Could you check a few things on this drawing? It's one solid part, dimensions in mm from its lowest x, y, z. Give positions to 0.01 mm unless a question says otherwise; leave off trailing zeros. Loops run counter-clockwise (first coordinate to the right, second up) from the corner with the lowest first, then second, coordinate; pieces in that order, holes last. Notation, with made-up numbers: (38.25, 69.25) - (66.25, 69.25) arc R8 ccw to (66.25, 74.25) - close; hole circle Ø11 at (66.25, 21.25). An arc over 180 degrees is marked (long way). Answer as a JSON object with one key per item and string values.
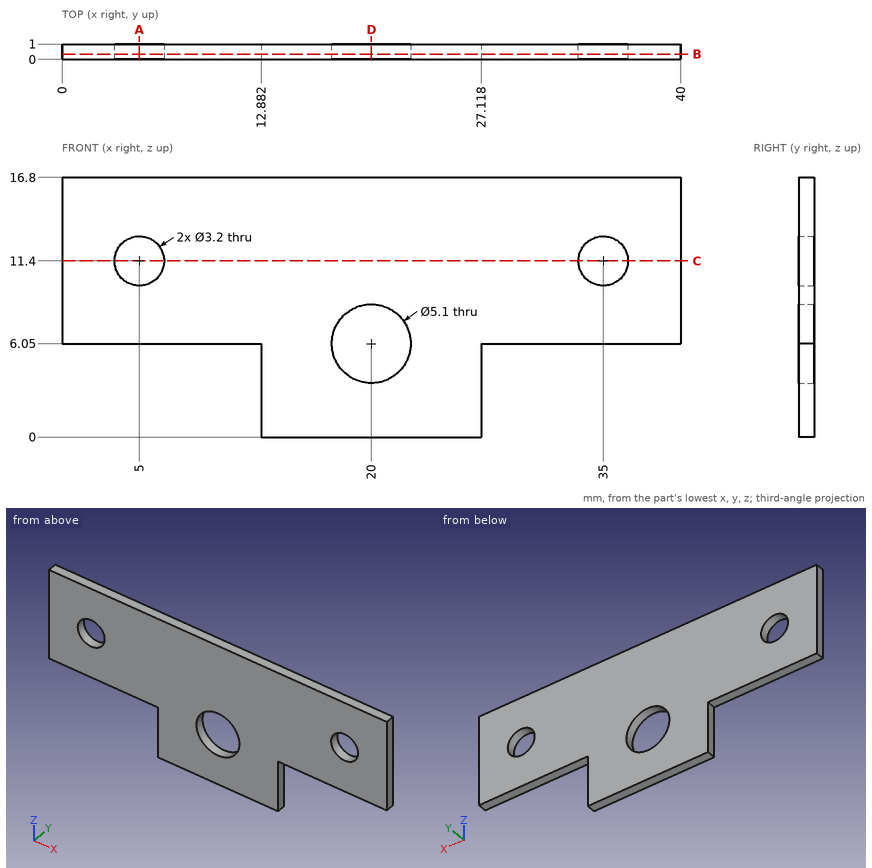
1) Imagine slicing it at B-B on y = 0.35. Write out the boundary of the cut face in (x, z).
Check sheet entries:
{"outline": "(0, 6.05) - (12.88, 6.05) - (12.88, 0) - (27.12, 0) - (27.12, 6.05) - (40, 6.05) - (40, 16.8) - (0, 16.8) - close; hole circle Ø3.2 at (5, 11.4); hole circle Ø5.1 at (20, 6.05); hole circle Ø3.2 at (35, 11.4)"}
2) Imagine slicing it at D-D on x = 20. Write out the boundary of the cut face in (y, z).
Check sheet entries:
{"outline": "(0, 0) - (1, 0) - (1, 3.5) - (0, 3.5) - close; (0, 8.6) - (1, 8.6) - (1, 16.8) - (0, 16.8) - close"}
3) I'm going to push a flat-ended pin straight in: P1, Ø0.5, axis at x = 4.5, y = 0.5, coming from the -Z side. Where does the tip first touch, or does it pass through?
Check sheet entries:
{"P1": "z = 6.05"}
4) Imagine slicing it at A-A on x = 5. Write out the boundary of the cut face in (y, z).
Check sheet entries:
{"outline": "(0, 6.05) - (1, 6.05) - (1, 9.8) - (0, 9.8) - close; (0, 13) - (1, 13) - (1, 16.8) - (0, 16.8) - close"}
5) I need wall thicknesses on L1, parallel to X at y = 0.5, z = 11.4; L2, parallel to Z at x = 35, y = 0.4; L3, parallel to Z at x = 7.5, y = 0.45. Which ranges of each line are inside material? Lowest first, please.
Check sheet entries:
{"L1": "0 to 3.4, 6.6 to 33.4, 36.6 to 40", "L2": "6.05 to 9.8, 13 to 16.8", "L3": "6.05 to 16.8"}
6) Imagine slicing it at C-C on z = 11.4. Write out the boundary of the cut face in (x, y).
Check sheet entries:
{"outline": "(0, 0) - (3.4, 0) - (3.4, 1) - (0, 1) - close; (6.6, 0) - (33.4, 0) - (33.4, 1) - (6.6, 1) - close; (36.6, 0) - (40, 0) - (40, 1) - (36.6, 1) - close"}
